The listing builds one solid part. Answer for the finished solid, in the listing's coordinates (mm). Face numbers are marked on the shaded views. A direction names the side the tool comes from. Coordinates: 2 decimals unless noted, no trailing zeros. Write each loop counter-clockwise with the first axis right and the second up, starting at its lowest first coordinate (ties: lowest second). Pieces come first, ordered by that corner, then holes. Notation, with made-up numbers: M 70.25,47.25 L 123.25,47.25 A8 ccw 123.25,59.25 Z; hole C 41,86.25 d8. An arc over 180 degrees is marked long. Answer as a JSON object with one key per item and string values. Group by question number.
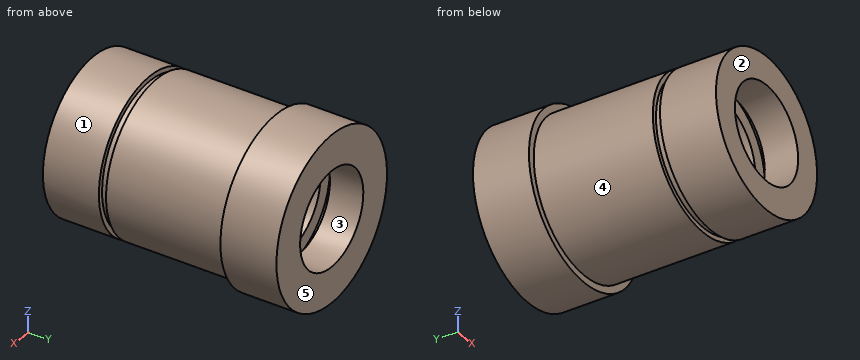
from build123d import *

# Parameters (mm, degrees)
SKETCH2_R          = 10
CUT_EXTRUDE1_DEPTH = 56.789784011
SKETCH3_R          = 13
CUT_EXTRUDE2_DEPTH = 2
CUT_EXTRUDE3_START = -2
SKETCH4_R          = 13
CUT_EXTRUDE3_DEPTH = 2


with BuildPart() as part:
    # Sketch1 → Revolve1 (revolve)
    with BuildSketch(Plane.XY, mode=Mode.PRIVATE) as revolve1_sk:
        Polygon((0, 23.132117765), (17.5, 23.132117765), (17.5, 11.382117765), (16, 11.382117765), (16, -13.617882235), (15, -13.617882235), (15, -15.117882235), (16, -15.117882235), (16, -26.867882235), (0, -26.867882235), align=None)
    revolve(revolve1_sk.sketch.rotate(Axis((0, 23.362720403, 0), (0, -1, 0)), 90), axis=Axis((0, 23.362720403, 0), (0, -1, 0)))

    # Sketch2 → Cut-Extrude1 (cut, through all)
    with BuildSketch(Plane(origin=(0, 23.132117765, 0), x_dir=(1, 0, 0), z_dir=(0, 1, 0))):
        with Locations(Location((0, 0, 0), (0, 0, 270))):
            Circle(SKETCH2_R)
    extrude(amount=-CUT_EXTRUDE1_DEPTH, mode=Mode.SUBTRACT)

    # Sketch3 → Cut-Extrude2 (cut)
    with BuildSketch(Plane(origin=(0, 16.132117765, 0), x_dir=(1, 0, 0), z_dir=(0, 1, 0))):
        with Locations(Location((0, 0, 0), (0, 0, 270))):
            Circle(SKETCH3_R)
    extrude(amount=-CUT_EXTRUDE2_DEPTH, mode=Mode.SUBTRACT)

    # Sketch4 → Cut-Extrude3 (cut)
    with BuildSketch(Plane(origin=(0, -19.867882235, 0), x_dir=(-1, 0, 0), z_dir=(0, -1, 0)).offset(CUT_EXTRUDE3_START)):
        with Locations(Location((0, 0, 0), (0, 0, 270))):
            Circle(SKETCH4_R)
    extrude(amount=CUT_EXTRUDE3_DEPTH, mode=Mode.SUBTRACT)


solid = part.part
Item 1: Consider L1, parallel to Y at x = 9.5, z = 6.5; L2, parallel to X at y = -18.7, z = 0; L3, parallel to Y at x = -5.5, z = -14. Determine where each line is inside the solid, lowest interval first. Write a range as from..to.
Item 2: A cutting plane is placed at C-C, the plane y = -9.5. Write down the section's boundary in (x, z), and give its area (3 significant figures).
Item 3: A tool of negligible diameter and unlimited length cuts with its end or side. For the marked faces 4 and 5, from which of +Z, -Z, +X, -X, +Y, -Y can it reach the whole face along a straight path? Write none if from no direction.
Item 4: For a pull along X with two mould halves and no side action, classify the marked faces 1, 2 and 3 as +X half, -X half, draft (parallel to the pull), parting line (faces both ways), or undercut.
Item 5: Flat-ended cylindrical pins translate along their axes: pin 1 Ø6 at (y, z) = (13.5, 10) entering from -X; pin 2 Ø4 at (y, z) = (-7, 8) entering from -X; pin 3 Ø6 at (x, y) = (-3, -4) entering from -Z. Find the tip coordinate at first contact, or state that the pin passes through.
Item 6: A cutting plane is placed at B-B, the plane z = 14. Write down the section's boundary in (x, y), and give its area (3 significant figures).
Item 7: A cutting plane is placed at A-A, the plane y = 15.5. Write down the section's boundary in (x, z).
Answer:
{
 "1": {"L1": "-26.87..-19.87, -17.87..14.13, 16.13..23.13", "L2": "-16..-13, 13..16", "L3": "-26.87..-15.12, -13.62..23.13"},
 "2": {"outline": "C 0,0 d32; hole C 0,0 d20", "area": "490 mm2"},
 "3": {"face 4": "-Y", "face 5": "+Z, -Z, +X, -X, +Y"},
 "4": {"face 1": "parting line", "face 2": "draft", "face 3": "undercut"},
 "5": {"pin 1": "x = -16.04", "pin 2": "x = -14.83", "pin 3": "z = -16"},
 "6": {"outline": "M -10.5,11.38 L -7.75,11.38 L -7.75,-13.62 L -5.39,-13.62 L -5.39,-15.12 L -7.75,-15.12 L -7.75,-26.87 L 7.75,-26.87 L 7.75,-15.12 L 5.39,-15.12 L 5.39,-13.62 L 7.75,-13.62 L 7.75,11.38 L 10.5,11.38 L 10.5,23.13 L -10.5,23.13 Z", "area": "832 mm2"},
 "7": {"outline": "C 0,0 d35; hole C 0,0 d26"}
}
